```python
from build123d import *

# Parameters (mm, degrees)
SKETCH1_W           = 153
SKETCH1_H           = 18
BOSS_EXTRUDE1_DEPTH = 12
BOSS_EXTRUDE2_START = -12
SKETCH2_W           = 12
SKETCH2_H           = 18
BOSS_EXTRUDE2_DEPTH = 40
BOSS_EXTRUDE3_START = -12
SKETCH3_R           = 9
BOSS_EXTRUDE3_DEPTH = 13
SKETCH4_R           = 7.4
CUT_EXTRUDE1_DEPTH  = 11.4
SKETCH5_R           = 1.6
CUT_EXTRUDE2_DEPTH  = 172.871347234
CUT_EXTRUDE4_START  = -11.4
SKETCH9_R           = 7.4
CUT_EXTRUDE4_DEPTH  = 11.4
FILLET1_R           = 20
FILLET2_R           = 5
FILLET3_R           = 2


with BuildPart() as part:
    # Sketch1 → Boss-Extrude1 (new body)
    with BuildSketch(Plane.XY):
        Rectangle(SKETCH1_W, SKETCH1_H)
    extrude(amount=BOSS_EXTRUDE1_DEPTH)

    # Sketch2 → Boss-Extrude2 (add)
    with BuildSketch(Plane(origin=(0, 0, 0), x_dir=(-1, 0, 0), z_dir=(0, 0, -1)).offset(BOSS_EXTRUDE2_START)):
        with Locations((82.5, 0)):
            Rectangle(SKETCH2_W, SKETCH2_H)
    boss_extrude2 = extrude(amount=BOSS_EXTRUDE2_DEPTH)

    # Sketch3 → Boss-Extrude3 (add)
    with BuildSketch(Plane.ZY.offset(88.5).offset(BOSS_EXTRUDE3_START)):
        with Locations((-28, 0)):
            Circle(SKETCH3_R)
    boss_extrude3 = extrude(amount=BOSS_EXTRUDE3_DEPTH)

    # Mirror1: Boss-Extrude2, Boss-Extrude3 across plane
    add(boss_extrude2.mirror(Plane(origin=(0, 0, 0), x_dir=(0, 0, 1), z_dir=(1, 0, 0))))
    add(boss_extrude3.mirror(Plane(origin=(0, 0, 0), x_dir=(0, 0, 1), z_dir=(1, 0, 0))))

    # Sketch4 → Cut-Extrude1 (cut)
    with BuildSketch(Plane.ZY.offset(89.5)):
        with Locations((-28, 0)):
            Circle(SKETCH4_R)
    extrude(amount=-CUT_EXTRUDE1_DEPTH, mode=Mode.SUBTRACT)

    # Sketch5 → Cut-Extrude2 (cut, through all)
    with BuildSketch(Plane.ZY.offset(78.1)):
        with Locations((-28, 0)):
            Circle(SKETCH5_R)
    extrude(amount=-CUT_EXTRUDE2_DEPTH, mode=Mode.SUBTRACT)

    # Sketch9 → Cut-Extrude4 (cut)
    with BuildSketch(Plane(origin=(89.5, 0, 0), x_dir=(0, 0, -1), z_dir=(1, 0, 0)).offset(CUT_EXTRUDE4_START)):
        with Locations(Location((28, 0, 0), (0, 0, 180))):
            Circle(SKETCH9_R)
    extrude(amount=CUT_EXTRUDE4_DEPTH, mode=Mode.SUBTRACT)

    # Fillet1
    fillet1_edges = [part.edges().sort_by_distance(p)[0] for p in [
        (-88.5, 0, 12),
        (88.5, 0, 12),
    ]]
    fillet(fillet1_edges, radius=FILLET1_R)

    # Fillet2
    fillet2_edges = [part.edges().sort_by_distance(p)[0] for p in [
        (76.5, 0, 0),
        (-76.5, 0, 0),
    ]]
    fillet(fillet2_edges, radius=FILLET2_R)

    # Fillet3
    # the kernel refuses this fillet: 2 mm, written as the material it takes off along each edge
    with BuildSketch(Plane(origin=(-76.5, 0, -28), x_dir=(0, 1, 0), z_dir=(0, 0, 1))) as fillet3_piece_1:
        with BuildLine():
            CenterArc((9 - FILLET3_R, FILLET3_R), FILLET3_R, 270, 90)
            Line((9, FILLET3_R), (9, 0))
            Line((9, 0), (9 - FILLET3_R, 0))
        make_face()
    revolve(axis=Axis((-76.5, 0, -28), (-1, 0, 0)), revolution_arc=180, mode=Mode.SUBTRACT)
    with BuildSketch(Plane(origin=(76.5, 0, -28), x_dir=(0, 1, 0), z_dir=(0, 0, 1))) as fillet3_piece_2:
        with BuildLine():
            CenterArc((9 - FILLET3_R, -FILLET3_R), FILLET3_R, 0, 90)
            Line((9, -FILLET3_R), (9, 0))
            Line((9, 0), (9 - FILLET3_R, 0))
        make_face()
    revolve(axis=Axis((76.5, 0, -28), (-1, 0, 0)), revolution_arc=180, mode=Mode.SUBTRACT)
    with BuildSketch(Plane(origin=(68.5, 9, 12), x_dir=(0, -1, 0), z_dir=(-1, 0, 0)), Plane(origin=(68.5, -9, 12), x_dir=(0, 0, -1), z_dir=(-1, 0, 0))) as fillet3_piece_3:
        with BuildLine():
            CenterArc((FILLET3_R, -FILLET3_R), FILLET3_R, 90, 90)
            Line((0, -FILLET3_R), (0, 0))
            Line((0, 0), (FILLET3_R, 0))
        make_face()
    extrude(amount=137, mode=Mode.SUBTRACT)
    with BuildSketch(Plane(origin=(-88.5, 9, -8), x_dir=(0, -1, 0), z_dir=(0, 0, -1))) as fillet3_piece_4_section:
        with BuildLine():
            CenterArc((FILLET3_R, -FILLET3_R), FILLET3_R, 90, 90)
            Line((0, -FILLET3_R), (0, 0))
            Line((0, 0), (FILLET3_R, 0))
        make_face()
    fillet3_piece_4 = extrude(amount=25, mode=Mode.PRIVATE)
    fillet3_piece_4 = fillet3_piece_4 - Plane(origin=(-88.080537714, 0, -28), x_dir=(0, 0, 1), z_dir=(1, 0, 0)) * Cylinder(9, 59, mode=Mode.PRIVATE)
    add(fillet3_piece_4, mode=Mode.SUBTRACT)
    with BuildSketch(Plane(origin=(88.5, 9, -8), x_dir=(0, -1, 0), z_dir=(0, 0, -1))) as fillet3_piece_5_section:
        with BuildLine():
            CenterArc((FILLET3_R, FILLET3_R), FILLET3_R, 180, 90)
            Line((0, FILLET3_R), (0, 0))
            Line((0, 0), (FILLET3_R, 0))
        make_face()
    fillet3_piece_5 = extrude(amount=25, mode=Mode.PRIVATE)
    fillet3_piece_5 = fillet3_piece_5 - Plane(origin=(88.080537714, 0, -28), x_dir=(0, 0, 1), z_dir=(-1, 0, 0)) * Cylinder(9, 59, mode=Mode.PRIVATE)
    add(fillet3_piece_5, mode=Mode.SUBTRACT)
    with BuildSketch(Plane(origin=(-68.5, 9, -8), x_dir=(-1, 0, 0), z_dir=(0, 0, -1))) as fillet3_piece_6:
        with BuildLine():
            CenterArc((20 - FILLET3_R, -FILLET3_R), FILLET3_R, 0, 90)
            Line((20 - FILLET3_R, 0), (20, 0))
            Line((20, 0), (20, -FILLET3_R))
        make_face()
    revolve(axis=Axis((-68.5, 9, -8), (0, 1, 0)), revolution_arc=90, mode=Mode.SUBTRACT)
    with BuildSketch(Plane(origin=(68.5, 9, -8), x_dir=(1, 0, 0), z_dir=(0, 0, -1))) as fillet3_piece_7:
        with BuildLine():
            CenterArc((20 - FILLET3_R, FILLET3_R), FILLET3_R, 270, 90)
            Line((20 - FILLET3_R, 0), (20, 0))
            Line((20, 0), (20, FILLET3_R))
        make_face()
    revolve(axis=Axis((68.5, 9, -8), (0, -1, 0)), revolution_arc=90, mode=Mode.SUBTRACT)
    with BuildSketch(Plane(origin=(88.5, -9, -8), x_dir=(-1, 0, 0), z_dir=(0, 0, -1))) as fillet3_piece_8_section:
        with BuildLine():
            CenterArc((FILLET3_R, FILLET3_R), FILLET3_R, 180, 90)
            Line((0, FILLET3_R), (0, 0))
            Line((0, 0), (FILLET3_R, 0))
        make_face()
    fillet3_piece_8 = extrude(amount=25, mode=Mode.PRIVATE)
    fillet3_piece_8 = fillet3_piece_8 - Plane(origin=(87.881585808, 0, -28), x_dir=(0, 0, 1), z_dir=(-1, 0, 0)) * Cylinder(9, 59, mode=Mode.PRIVATE)
    add(fillet3_piece_8, mode=Mode.SUBTRACT)
    with BuildSketch(Plane(origin=(-88.5, -9, -8), x_dir=(1, 0, 0), z_dir=(0, 0, -1))) as fillet3_piece_9_section:
        with BuildLine():
            CenterArc((FILLET3_R, -FILLET3_R), FILLET3_R, 90, 90)
            Line((0, -FILLET3_R), (0, 0))
            Line((0, 0), (FILLET3_R, 0))
        make_face()
    fillet3_piece_9 = extrude(amount=25, mode=Mode.PRIVATE)
    fillet3_piece_9 = fillet3_piece_9 - Plane(origin=(-87.881599188, 0, -28), x_dir=(0, 0, 1), z_dir=(1, 0, 0)) * Cylinder(9, 59, mode=Mode.PRIVATE)
    add(fillet3_piece_9, mode=Mode.SUBTRACT)
    with BuildSketch(Plane(origin=(-68.5, -9, -8), x_dir=(-1, 0, 0), z_dir=(0, 0, -1))) as fillet3_piece_10:
        with BuildLine():
            CenterArc((20 - FILLET3_R, FILLET3_R), FILLET3_R, 270, 90)
            Line((20, FILLET3_R), (20, 0))
            Line((20, 0), (20 - FILLET3_R, 0))
        make_face()
    revolve(axis=Axis((-68.5, -9, -8), (0, 1, 0)), revolution_arc=90, mode=Mode.SUBTRACT)
    with BuildSketch(Plane(origin=(68.5, -9, -8), x_dir=(1, 0, 0), z_dir=(0, 0, -1))) as fillet3_piece_11:
        with BuildLine():
            CenterArc((20 - FILLET3_R, -FILLET3_R), FILLET3_R, 0, 90)
            Line((20, -FILLET3_R), (20, 0))
            Line((20, 0), (20 - FILLET3_R, 0))
        make_face()
    revolve(axis=Axis((68.5, -9, -8), (0, -1, 0)), revolution_arc=90, mode=Mode.SUBTRACT)
    with BuildSketch(Plane(origin=(-76.5, -9, -5), x_dir=(-1, 0, 0), z_dir=(0, 0, -1)), Plane(origin=(-76.5, 9, -5), x_dir=(0, -1, 0), z_dir=(0, 0, -1))) as fillet3_piece_12:
        with BuildLine():
            CenterArc((FILLET3_R, FILLET3_R), FILLET3_R, 180, 90)
            Line((0, FILLET3_R), (0, 0))
            Line((0, 0), (FILLET3_R, 0))
        make_face()
    extrude(amount=23, mode=Mode.SUBTRACT)
    with BuildSketch(Plane(origin=(-71.5, 9, 0), x_dir=(0, -1, 0), z_dir=(1, 0, 0))) as fillet3_piece_13:
        with BuildLine():
            CenterArc((FILLET3_R, -FILLET3_R), FILLET3_R, 90, 90)
            Line((0, -FILLET3_R), (0, 0))
            Line((0, 0), (FILLET3_R, 0))
        make_face()
    extrude(amount=143, mode=Mode.SUBTRACT)
    with BuildSketch(Plane(origin=(71.5, -9, 0), x_dir=(0, 0, 1), z_dir=(-1, 0, 0))) as fillet3_piece_14:
        with BuildLine():
            CenterArc((FILLET3_R, FILLET3_R), FILLET3_R, 180, 90)
            Line((0, FILLET3_R), (0, 0))
            Line((0, 0), (FILLET3_R, 0))
        make_face()
    extrude(amount=143, mode=Mode.SUBTRACT)
    with BuildSketch(Plane(origin=(76.5, 9, -5), x_dir=(0, -1, 0), z_dir=(0, 0, -1)), Plane(origin=(76.5, -9, -5), x_dir=(1, 0, 0), z_dir=(0, 0, -1))) as fillet3_piece_15:
        with BuildLine():
            CenterArc((FILLET3_R, -FILLET3_R), FILLET3_R, 90, 90)
            Line((0, -FILLET3_R), (0, 0))
            Line((0, 0), (FILLET3_R, 0))
        make_face()
    extrude(amount=23, mode=Mode.SUBTRACT)
    with BuildSketch(Plane(origin=(-71.5, -9, -5), x_dir=(-1, 0, 0), z_dir=(0, 0, -1))) as fillet3_piece_16:
        with BuildLine():
            CenterArc((5 + FILLET3_R, FILLET3_R), FILLET3_R, 180, 90)
            Line((5, FILLET3_R), (5, 0))
            Line((5, 0), (5 + FILLET3_R, 0))
        make_face()
    revolve(axis=Axis((-71.5, -9, -5), (0, 1, 0)), revolution_arc=90, mode=Mode.SUBTRACT)
    with BuildSketch(Plane(origin=(-71.5, 9, -5), x_dir=(-1, 0, 0), z_dir=(0, 0, -1))) as fillet3_piece_17:
        with BuildLine():
            CenterArc((5 + FILLET3_R, -FILLET3_R), FILLET3_R, 90, 90)
            Line((5 + FILLET3_R, 0), (5, 0))
            Line((5, 0), (5, -FILLET3_R))
        make_face()
    revolve(axis=Axis((-71.5, 9, -5), (0, 1, 0)), revolution_arc=90, mode=Mode.SUBTRACT)
    with BuildSketch(Plane(origin=(71.5, 9, -5), x_dir=(0, 0, 1), z_dir=(-1, 0, 0))) as fillet3_piece_18:
        with BuildLine():
            CenterArc((5 + FILLET3_R, -FILLET3_R), FILLET3_R, 90, 90)
            Line((5 + FILLET3_R, 0), (5, 0))
            Line((5, 0), (5, -FILLET3_R))
        make_face()
    revolve(axis=Axis((71.5, 9, -5), (0, 1, 0)), revolution_arc=90, mode=Mode.SUBTRACT)
    with BuildSketch(Plane(origin=(71.5, -9, -5), x_dir=(0, 0, 1), z_dir=(-1, 0, 0))) as fillet3_piece_19:
        with BuildLine():
            CenterArc((5 + FILLET3_R, FILLET3_R), FILLET3_R, 180, 90)
            Line((5, FILLET3_R), (5, 0))
            Line((5, 0), (5 + FILLET3_R, 0))
        make_face()
    revolve(axis=Axis((71.5, -9, -5), (0, 1, 0)), revolution_arc=90, mode=Mode.SUBTRACT)


solid = part.part
```
Verification items for the finished model (mm, model axes). A direction names the side the tool comes from. Round coordinates to 2 decimals unless told otherwise and drop trailing zeros. Order: outer loops, then holes, each group sorted by start corner. A loop starts at its lowest first (then second) coordinate and runs counter-clockwise, first axis right, second up.
1) Tool access check on faces 1 (the cylindrical face through (-83.88, 0.325, -35.393)), 2 (the cylindrical face through (83.72, 4.503, -33.872)), 3 (the flat face through (76.5, 0, -20)), 4 (the cylindrical face through (-77.31, 1.08, -29.18)), 5 (the flat face through (-89.5, -7.3, -30)). Record the directions out of +Z, -Z, +X, -X, +Y, -Y that give a thin tool (end or side, any length) a straight path to the whole face; none if there is none.
Geometry says:
face 1: -X
face 2: +X
face 3: -Z, +Y, -Y
face 4: +X, -X
face 5: +Z, -Z, -X, +Y, -Y
2) Material ranges on line 1 (X direction, y = 6.75, z = -29); line 2 (X direction, y = -4, z = -12.5); line 3 (Y direction, x = -77.25, z = -28), recorded low to high.
Geometry says:
line 1: x = -78.1 to -76.5, 76.5 to 78.1
line 2: x = -88.5 to -76.5, 76.5 to 88.5
line 3: y = -8.56 to -1.6, 1.6 to 8.56
3) Cross-section at A-A, the plane y = 0. Give the number of separate pieces and of enclosed holes in the cut face, plus the area to 3 significant figures.
Geometry says:
separate pieces: 3
enclosed holes: 0
area: 2,540 mm2
4) Depth check by flat-ended pin: pin 1 (9 mm diameter, centred on y = 0, z = -28, fed in from +X); pin 2 (4 mm diameter, centred on x = -16.5, y = 0, fed in from -Z); pin 3 (7.5 mm diameter, centred on y = -2.5, z = -25.5, fed in from -X). Enter the tip coordinate at first touch or a pass-through.
Geometry says:
pin 1: stops at x = 78.1
pin 2: stops at z = 0
pin 3: stops at x = -78.1
5) Cross-section at B-B, the plane x = 57. Record the cut outline in (y, z).
Geometry says:
outline: (-9, 2) arc R2 ccw to (-7, 0) - (7, 0) arc R2 ccw to (9, 2) - (9, 10) arc R2 ccw to (7, 12) - (-7, 12) arc R2 ccw to (-9, 10) - close
6) Draft check along Y on faces 6 (the flat face through (-78.1, 2, -28)), 7 (the flat face through (0, -9, 4)), 8 (the cylindrical face through (75.07, 0.1, -1.5)). Enter one of: +Y half, -Y half, draft (parallel to the pull), parting line (faces both ways), or undercut.
Geometry says:
face 6: undercut
face 7: -Y half
face 8: draft
